Geometry: final body of the model. Coordinates: model frame, mm. Face numbers are marked on the shaded views. A direction names the side the tool comes from. Round coordinates to 2 decimals unless told otherwise and drop trailing zeros. Write each loop counter-clockwise with the first axis right and the second up, starting at its lowest first coordinate (ties: lowest second). Pieces come first, ordered by that corner, then holes. Notation, with made-up numbers: (31, 29) -> (38, 29) arc R13 ccw to (38, 44) -> close; hole circle Ø3 at (70.25, 81.5). An arc over 180 degrees is marked (long way). Use one line per item in the form item = value. Start each with the question number.
1. Cut plane B-B, the plane x = 3. Return the cut outline in (y, z), plus the area to 3 significant figures.
2. Reachability of the marked faces 4 and 5 from +Z, -Z, +X, -X, +Y, -Y: full face, straight path, thin tool, end or side. Return the list, or none.
3. Pin query (flat end, axial travel): pin 1 Ø5 at (x, y) = (9.5, 33) entering from -Z; pin 2 Ø4 at (x, z) = (33.5, -27) entering from -Y; pin 3 Ø2.5 at (y, z) = (-26, -1) entering from +X; pin 4 Ø14.5 at (y, z) = (-28.99, -28.99) entering from -X. Return the tip coordinate at first contact, or that it passes through.
4. Line query: L1, parallel to X at y = 24.5, z = 34.5; L2, parallel to Y at x = 24, z = 8; L3, parallel to Y at x = 32.5, z = 17. Output: solid intervals per line, ascending.
5. Draft query along Z for the marked faces 1, 2 and 3. Return one class per face: pulls with the +Z half, pulls with the -Z half, needs draft (parallel to the pull), parting line crosses it, or undercut.
6. Cut plane A-A, the plane z = 0. Return the cut outline in (x, y), plus the area to 3 significant figures.
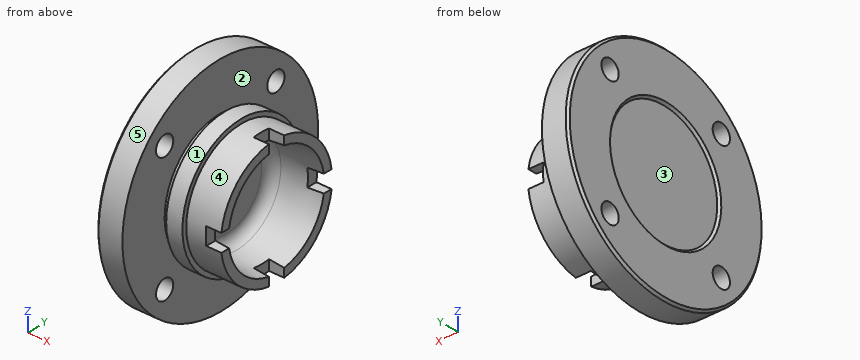
Autodesk Inventor part; units mm, degrees
ref_plane "YZ Plane" through (0, 0, 0) normal (1, 0, 0) x (0, 1, 0)
ref_plane "XZ Plane" through (0, 0, 0) normal (0, 1, 0) x (-1, 0, 0)
ref_plane "XY Plane" through (0, 0, 0) normal (0, 0, 1) x (1, 0, 0)
sketch "草图1" plane through (0, 0, 0) normal (0, 1, 0) x (-1, 0, 0)
  line L0 (0, 51) -> (-12, 51)
  line L1 (-12, 51) -> (-12, 29)
  line L2 (-12, 29) -> (-14.5, 29)
  line L3 (-14.5, 29) -> (-14.5, 31)
  line L4 (-14.5, 31) -> (-22, 31)
  line L5 (-22, 31) -> (-22, 29)
  line L6 (-22, 29) -> (-38, 29)
  line L7 (-38, 29) -> (-38, 0)
  line L8 (-38, 0) -> (0, 0)
  line L9 (0, 0) -> (0, 51)
  line L10 (0, 29) -> (-1, 28)
  line L11 (-1, 28) -> (-1, 0)
  line L12 (-38, 25) -> (-15, 22.6998)
  line L13 (-15, 22.6998) -> (-15, 0)
  line L14 (7.6, 0) -> (-45.6, 0)
  dimension "d2" = 51
  dimension "d4" = 26
  dimension "d5" = 12
  dimension "d6" = 31
  dimension "d7" = 29
  dimension "d8" = 10
  dimension "d9" = 2.5
  dimension "d10" = 29
  dimension "d11" = 45
  dimension "d12" = 1
  dimension "d13" = 15
  dimension "d14" = 25
  dimension "d15" = 84.289
revolve "旋转1" add sketch "草图1" angle 360 about axis through (-10, 0, 0) along (1, 0, 0) contours L9 L10 L11 L8 L13 L12 L7 L6 L5 L4 L3 L2 L1 L0
sketch "草图2" plane through (0, 0, 0) normal (0, 1, 0) x (-1, 0, 0)
  line L0 (-22, 29) -> (-38, 29)
  line L1 (-38, 29) -> (-31, 29)
  line L2 (-31, 29) -> (-31, -29)
  line L3 (-31, -29) -> (-38, -29)
  line L4 (-38, -29) -> (-38, 29)
  point P0 (0, 0)
  dimension "d17" = 7
extrude "拉伸1" cut sketch "草图2" along normal mid plane 8
sketch "草图3" plane through (0, 0, 0) normal (0, 0, 1) x (1, 0, 0)
  line L0 (38, 4) -> (38, 29)
  line L1 (22, -29) -> (38, -29)
  line L2 (38, 29) -> (31, 29)
  line L3 (31, 29) -> (31, -29)
  line L4 (31, -29) -> (38, -29)
  line L5 (38, -29) -> (38, 29)
  point P0 (0, 0)
  dimension "d20" = 7
extrude "拉伸2" cut sketch "草图3" along normal mid plane 8
sketch "草图4" plane through (0, 0, 0) normal (-1, 0, 0) x (0, 0, 1)
  circle A0 centre (28.9914, 28.9914) radius 4.5
  circle A1 centre (-28.9914, 28.9914) radius 4.5
  circle A2 centre (-28.9914, -28.9914) radius 4.5
  circle A3 centre (28.9914, -28.9914) radius 4.5
  line L0 (28.9914, 28.9914) -> (0, 0)
  line L1 (0, -71.4) -> (0, 71.4)
  dimension "d23" = 9
  dimension "d24" = 41
  dimension "d27" = 360
  dimension "d35" = 45
extrude "拉伸3" cut sketch "草图4" against normal up to surface (12 mm away)
chamfer "倒角1" distance 1 angle 45 1 edges at (0, 0, -51)
fillet "圆角1" radius 5 1 edges at (15, 0, -22.6998)
equation "\"d2\" = 0.5 * D2"
equation "\"d4\" = M"
equation "\"d5\" = e"
equation "\"d6\" = 0.5 * D"
equation "\"d7\" = 0.5 * D_d"
equation "\"d8\" = e1"
equation "\"d10\" = 0.5 * D_d"
equation "\"d13\" = b1"
equation "\"d14\" = 0.5 * D4"
equation "\"d17\" = h_b"
equation "\"d18\" = b"
equation "\"d20\" = h_b"
equation "\"d21\" = b"
equation "\"d23\" = d0"
equation "\"d24\" = 0.5 * D0"
equation "\"d29\" = b"
equation "\"d3\" = 8"
equation "\"d0\" = 9"
equation "\"D\" = 62"
equation "\"D0\" = 82"
equation "\"D2\" = 102"
equation "\"D_d\" = 58"
equation "\"e\" = 12"
equation "\"e1\" = 10"
equation "\"b\" = 8"
equation "\"h_b\" = 7"
equation "\"M\" = 26"
equation "\"b1\" = 15"
equation "\"d1\" = 26"
properties part number "高速轴承闷盖" material "灰口铁"
Outcome:
q1.outline = circle Ø102 at (0, 0); hole circle Ø9 at (-28.99, -28.99); hole circle Ø9 at (-28.99, 28.99); hole circle Ø9 at (28.99, -28.99); hole circle Ø9 at (28.99, 28.99)
q1.area = 7,920 mm^2
q2.face_4 = +X
q2.face_5 = +X, -X
q3.pin_1 = -40.87
q3.pin_2 = -14.7
q3.pin_3 = 31
q3.pin_4 = 0
q4.L1 = 0 to 12
q4.L2 = -27.87 to -22.2, 22.2 to 27.87
q4.L3 = -23.49 to -17.57, 17.57 to 23.49
q5.face_1 = parting line crosses it
q5.face_2 = needs draft
q5.face_3 = undercut
q6.outline = (0, -50) -> (1, -51) -> (12, -51) -> (12, -29) -> (14.5, -29) -> (14.5, -31) -> (22, -31) -> (22, -29) -> (31, -29) -> (31, -24.3) -> (19.5, -23.15) arc R5 cw to (15, -18.17) -> (15, 18.17) arc R5 cw to (19.5, 23.15) -> (31, 24.3) -> (31, 29) -> (22, 29) -> (22, 31) -> (14.5, 31) -> (14.5, 29) -> (12, 29) -> (12, 51) -> (1, 51) -> (0, 50) -> (0, 29) -> (1, 28) -> (1, -28) -> (0, -29) -> close
q6.area = 1,550 mm^2
